Geometry check sheet. Reference: the model listing, model coordinates, mm. A direction names the side the tool comes from. Coordinates: 2 decimals unless noted, no trailing zeros. Write each loop counter-clockwise with the first axis right and the second up, starting at its lowest first coordinate (ties: lowest second). Pieces come first, ordered by that corner, then holes. Notation, with made-up numbers: (13.5, -34) -> (49.5, -34) arc R30 ccw to (49.5, -11) -> close; hole circle Ø8 at (9, 0). An arc over 180 degrees is marked (long way). Use a Markdown table: item, result.
```python
from build123d import *

# Parameters (mm, degrees)
ESTRUSIONE_ESTRUSIONE1_DEPTH   = 62
ESTRUSIONE_ESTRUSIONE1_2_DEPTH = 62
SCHIZZO2_W                     = 57
SCHIZZO2_H                     = 41
SCHIZZO2_R                     = 5.5
ESTRUSIONE_ESTRUSIONE2_DEPTH   = 2
SCHIZZO3_R                     = 7.5
SCHIZZO3_R_2                   = 5.5
ESTRUSIONE_ESTRUSIONE3_DEPTH   = 2
SMUSSO1_SIZE                   = 2
SCHIZZO4_W                     = 57
SCHIZZO4_H                     = 41
SCHIZZO4_R                     = 2.6
ESTRUSIONE_ESTRUSIONE4_DEPTH   = 2
RACCORDO1_R                    = 8


with BuildPart() as part:
    # Schizzo1 → Estrusione-Estrusione1 (new body)
    with BuildSketch(Plane.XY):
        with BuildLine():
            Line((-28.5, -20.5), (-28.5, 20.5))
            Line((-28.5, 20.5), (-25.5, 20.5))
            Line((-25.5, 20.5), (-25.5, 0))
            ThreePointArc((-25.5, 0), (-22.770338685, -11.478748894), (-15.165750888, -20.5))
            Line((-15.165750888, -20.5), (-28.5, -20.5))
        make_face()
    extrude(amount=ESTRUSIONE_ESTRUSIONE1_DEPTH)



with BuildPart() as body_2:
    # Schizzo1 → Estrusione-Estrusione1 2 (new body)
    with BuildSketch(Plane.XY):
        with BuildLine():
            Line((28.5, 20.5), (25.5, 20.5))
            Line((25.5, 20.5), (25.5, 0))
            ThreePointArc((25.5, 0), (22.770338685, -11.478748894), (15.165750888, -20.5))
            Line((15.165750888, -20.5), (28.5, -20.5))
            Line((28.5, -20.5), (28.5, 20.5))
        make_face()
    extrude(amount=ESTRUSIONE_ESTRUSIONE1_2_DEPTH)


with BuildPart() as part_1:
    add(part.part)

    add(body_2.part)  # Estrusione-Estrusione2 merges body 2
    # Schizzo2 → Estrusione-Estrusione2 (add)
    with BuildSketch(Plane.XY.offset(62)):
        Rectangle(SCHIZZO2_W, SCHIZZO2_H)
        Circle(SCHIZZO2_R, mode=Mode.SUBTRACT)
    extrude(amount=ESTRUSIONE_ESTRUSIONE2_DEPTH)

    # Schizzo3 → Estrusione-Estrusione3 (add)
    with BuildSketch(Plane.XY.offset(64)):
        Circle(SCHIZZO3_R)
        Circle(SCHIZZO3_R_2, mode=Mode.SUBTRACT)
    extrude(amount=ESTRUSIONE_ESTRUSIONE3_DEPTH)

    # Smusso1
    smusso1_edges = [part_1.edges().sort_by_distance(p)[0] for p in [
        (-7.5, 0, 64),
    ]]
    chamfer(smusso1_edges, length=SMUSSO1_SIZE - 0.0001)  # a hair under: the kernel refuses the full size

    # Schizzo4 → Estrusione-Estrusione4 (add)
    with BuildSketch(Plane(origin=(0, 0, 0), x_dir=(-1, 0, 0), z_dir=(0, 0, -1))):
        Rectangle(SCHIZZO4_W, SCHIZZO4_H)
        Circle(SCHIZZO4_R, mode=Mode.SUBTRACT)
    extrude(amount=ESTRUSIONE_ESTRUSIONE4_DEPTH)

    # Raccordo1
    raccordo1_edges = [part_1.edges().sort_by_distance(p)[0] for p in [
        (-28.5, -20.5, 31),
        (28.5, -20.5, 31),
    ]]
    fillet(raccordo1_edges, radius=RACCORDO1_R)


solid = part_1.part
```
Item 1: Section check B-B on x = 0. Count the separate pieces of the cut face and the enclosed holes in it, then the cut area to 3 significant figures.
Answer block:
| item | result |
|---|---|
| separate pieces | 4 |
| enclosed holes | 0 |
| area | 144 mm^2 |
Item 2: Section check D-D on x = -12. Record the boundary of the cut face in (y, z), then the cut area to 3 significant figures.
Answer block:
| item | result |
|---|---|
| outline | (-20.5, -2) -> (20.5, -2) -> (20.5, 0) -> (-20.5, 0) -> close; (-20.5, 62) -> (20.5, 62) -> (20.5, 64) -> (-20.5, 64) -> close |
| area | 164 mm^2 |
Item 3: Section check C-C on y = 15.5. Record the boundary of the cut face in (x, z).
Answer block:
| item | result |
|---|---|
| outline | (-28.5, -2) -> (28.5, -2) -> (28.5, 64) -> (-28.5, 64) -> close; hole (-25.5, 0) -> (25.5, 0) -> (25.5, 62) -> (-25.5, 62) -> close |
Item 4: Depth check by flat-ended pin: P1, Ø20.5, axis at x = -12.5, y = -8.5, coming from the +Z side; P2, Ø7, axis at x = 0, y = 0, coming from the +Z side; P3, Ø1, axis at x = -18.5, y = -16.5, coming from the +Z side. Enter the tip coordinate at first touch or a pass-through.
Answer block:
| item | result |
|---|---|
| P1 | stops at z = 66 |
| P2 | stops at z = 0 |
| P3 | stops at z = 64 |
Item 5: Tool access check on faces 1 (the flat face through (0, 5, -2)), 2 (the cylindrical face through (22.845, -11.33, 30.566)), 3 (the cylindrical face through (-1.19, -5.37, 63.97)). Record the directions out of +Z, -Z, +X, -X, +Y, -Y that give a thin tool (end or side, any length) a straight path to the whole face; none if there is none.
Answer block:
| item | result |
|---|---|
| face 1 | -Z, +X, -X, +Y, -Y |
| face 2 | +Y |
| face 3 | +Z |
Item 6: Thickness scan on L1, parallel to Z at x = -15, y = 5; L2, parallel to X at y = 8.5, z = 57; L3, parallel to Z at x = -1, y = 4.5. Record the ranges inside material, lowest first. Write a range as [from, to].
Answer block:
| item | result |
|---|---|
| L1 | z = [-2, 0], [62, 64] |
| L2 | x = [-28.5, -25.5], [25.5, 28.5] |
| L3 | z = [-2, 0] |
Item 7: Section check A-A on z = 15.5. Record the boundary of the cut face in (x, y), then the cut area to 3 significant figures.
Answer block:
| item | result |
|---|---|
| outline | (-28.5, -12.5) arc R8 ccw to (-20.5, -20.5) -> (-15.17, -20.5) arc R25.5 cw to (-25.5, 0) -> (-25.5, 20.5) -> (-28.5, 20.5) -> close; (15.17, -20.5) -> (20.5, -20.5) arc R8 ccw to (28.5, -12.5) -> (28.5, 20.5) -> (25.5, 20.5) -> (25.5, 0) arc R25.5 cw to start |
| area | 346 mm^2 |
Item 8: Mould release check, pull along Z, two halves, no side actions. Record for faces 4 (the cylindrical face through (-22.845, -11.33, 30.566)), 5 (the flat face through (-4, 4, 66)), 6 (the flat face through (28.5, 4, 31)): +Z half, -Z half, draft (parallel to the pull), parting line (faces both ways), or undercut.
Answer block:
| item | result |
|---|---|
| face 4 | undercut |
| face 5 | +Z half |
| face 6 | draft |
